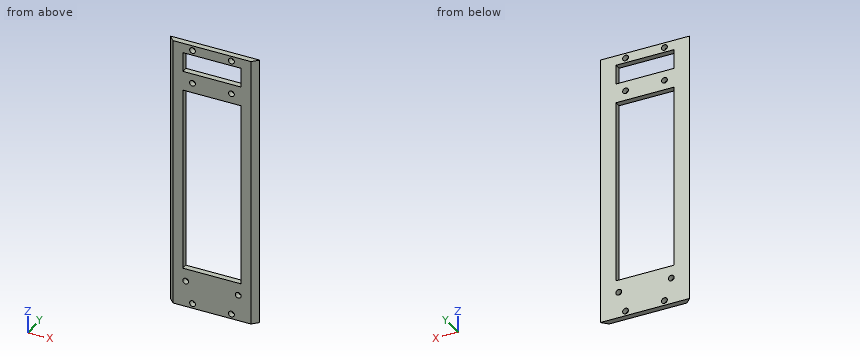
from build123d import *

# Parameters (mm, degrees)
SKETCH1_W           = 50
SKETCH1_H           = 140
BOSS_EXTRUDE2_DEPTH = 5
CUT_EXTRUDE1_DEPTH  = 152
SKETCH7_W           = 50
SKETCH7_H           = 2
CUT_EXTRUDE5_DEPTH  = 197
SKETCH8_W           = 30
SKETCH8_H           = 130
CUT_EXTRUDE6_DEPTH  = 197
SKETCH9_W           = 40
SKETCH9_H           = 20
SKETCH9_R           = 1.5
BOSS_EXTRUDE5_DEPTH = 3
SKETCH10_W          = 30
SKETCH10_H          = 10
SKETCH10_R          = 1.5
BOSS_EXTRUDE6_DEPTH = 3
SKETCH11_R          = 1.5
CUT_EXTRUDE7_DEPTH  = 3


with BuildPart() as part:
    # Sketch1 → Boss-Extrude2 (new body)
    with BuildSketch(Plane(origin=(0, 0, 0), x_dir=(1, 0, 0), z_dir=(0, 1, 0))):
        Rectangle(SKETCH1_W, SKETCH1_H)
    extrude(amount=BOSS_EXTRUDE2_DEPTH)

    # Sketch2 → Cut-Extrude1 (cut)
    with BuildSketch(Plane.XY.offset(70)):
        Polygon((-20, 0), (-25, 5), (-25, 0), align=None)
        Polygon((25, 5), (20, 0), (25, 0), align=None)
    extrude(amount=-CUT_EXTRUDE1_DEPTH, mode=Mode.SUBTRACT)

    # Sketch7 → Cut-Extrude5 (cut)
    with BuildSketch(Plane(origin=(0, 0, -70), x_dir=(-1, 0, 0), z_dir=(0, 0, -1))):
        with Locations((0, 4)):
            Rectangle(SKETCH7_W, SKETCH7_H)
    extrude(amount=-CUT_EXTRUDE5_DEPTH, mode=Mode.SUBTRACT)

    # Sketch8 → Cut-Extrude6 (cut)
    with BuildSketch(Plane.XZ):
        Rectangle(SKETCH8_W, SKETCH8_H)
    extrude(amount=-CUT_EXTRUDE6_DEPTH, mode=Mode.SUBTRACT)

    # Sketch9 → Boss-Extrude5 (add)
    with BuildSketch(Plane.XZ):
        with Locations((0, -60)):
            Rectangle(SKETCH9_W, SKETCH9_H)
        with Locations(Location((-13.5, -56.5, 0), (0, 0, 270))):
            Circle(SKETCH9_R, mode=Mode.SUBTRACT)
        with Locations(Location((13.5, -56.5, 0), (0, 0, 90))):
            Circle(SKETCH9_R, mode=Mode.SUBTRACT)
    extrude(amount=-BOSS_EXTRUDE5_DEPTH)

    # Sketch10 → Boss-Extrude6 (add)
    with BuildSketch(Plane.XZ):
        with Locations((0, 50)):
            Rectangle(SKETCH10_W, SKETCH10_H)
        with Locations(Location((-10, 50, 0), (0, 0, 270))):
            Circle(SKETCH10_R, mode=Mode.SUBTRACT)
        with Locations(Location((10, 50, 0), (0, 0, 270))):
            Circle(SKETCH10_R, mode=Mode.SUBTRACT)
    extrude(amount=-BOSS_EXTRUDE6_DEPTH)

    # Sketch11 → Cut-Extrude7 (cut)
    with BuildSketch(Plane.XZ):
        with Locations(Location((-10, 67.5, 0), (0, 0, 270))):
            Circle(SKETCH11_R)
        with Locations(Location((10, 67.5, 0), (0, 0, 90))):
            Circle(SKETCH11_R)
        with Locations(Location((10, -67.5, 0), (0, 0, 270))):
            Circle(SKETCH11_R)
        with Locations(Location((-10, -67.5, 0), (0, 0, 90))):
            Circle(SKETCH11_R)
    extrude(amount=-CUT_EXTRUDE7_DEPTH, mode=Mode.SUBTRACT)


solid = part.part
The listing builds one solid part. Answer for the finished solid, in the listing's coordinates (mm). Round coordinates to 2 decimals unless told otherwise and drop trailing zeros. Write each loop counter-clockwise with the first axis right and the second up, starting at its lowest first coordinate (ties: lowest second). Pieces come first, ordered by that corner, then holes. Notation, with made-up numbers: (-16.75, -10.5) - (-3.75, -10.5) arc R8 cw to (-3.75, 1.5) - close; hole circle Ø2 at (37, -27.5). An arc over 180 degrees is marked (long way). Use a Markdown table: item, result. Add a question column.
1. Consider line 1 (Z direction, x = -2.5, y = 0.2); line 2 (Z direction, x = 13.5, y = 1.5); line 3 (Z direction, x = 9, y = 2). Determine where each line is inside the solid, lowest interval first.
2. The part is cut by section C-C (y = 1.4). Give the number of separate pieces and of enclosed holes in the cut face, and give its area (3 significant figures).
3. The part is cut by section A-A (x = -13.5). Write down the section's boundary in (y, z).
4. The part is cut by section D-D (z = 38.5). Write down the section's boundary in (x, y).
5. Flat-ended cylindrical pins translate along their axes: P1, Ø0.9, axis at y = 1, z = 59, coming from the +X side; P2, Ø0.9, axis at y = 2, z = -8.5, coming from the -X side. Find the tip coordinate at first contact, or state that the pin passes through.
6. The part is cut by section B-B (z = -67.5). Write down the section's boundary in (x, y), and give its area (3 significant figures).
Reported:
| question | item | result |
|---|---|---|
| 1 | line 1 | -70 to -50, 45 to 55, 65 to 70 |
| 1 | line 2 | -70 to -58, -55 to -50, 45 to 55, 65 to 70 |
| 1 | line 3 | -70 to -68.62, -66.38 to -50, 45 to 48.88, 51.12 to 55, 65 to 66.38, 68.62 to 70 |
| 2 | separate pieces | 1 |
| 2 | enclosed holes | 10 |
| 2 | area | 2,790 mm^2 |
| 3 | outline | (0, -70) - (3, -70) - (3, -58) - (0, -58) - close; (0, -55) - (3, -55) - (3, -50) - (0, -50) - close; (0, 45) - (3, 45) - (3, 55) - (0, 55) - close; (0, 65) - (3, 65) - (3, 70) - (0, 70) - close |
| 4 | outline | (-23, 3) - (-20, 0) - (-15, 0) - (-15, 3) - close; (15, 0) - (20, 0) - (23, 3) - (15, 3) - close |
| 5 | P1 | x = 21.45 |
| 5 | P2 | x = -22.45 |
| 6 | outline | (-23, 3) - (-20, 0) - (-11.5, 0) - (-11.5, 3) - close; (-8.5, 0) - (8.5, 0) - (8.5, 3) - (-8.5, 3) - close; (11.5, 0) - (20, 0) - (23, 3) - (11.5, 3) - close |
| 6 | area | 111 mm^2 |
